Could you check a few things on this model? Use its own coordinates, in mm. A direction names the side the tool comes from. Give positions to 0.01 mm unless a question says otherwise; leave off trailing zeros. Write each loop counter-clockwise with the first axis right and the second up, starting at its lowest first coordinate (ties: lowest second). Pieces come first, ordered by that corner, then holes. Notation, with made-up numbers: M 72,3.25 L 124,3.25 A14 cw 124,28.25 Z; hole C 59.25,31.5 d3. An arc over 180 degrees is marked long. Use one line per item in the form item = value.
from build123d import *

# Parameters (mm, degrees)
SKETCH1_W           = 20.05
SKETCH1_H           = 21.2
BOSS_EXTRUDE1_DEPTH = 7
SKETCH2_W           = 20.05
SKETCH2_H           = 21.2
BOSS_EXTRUDE2_DEPTH = 1
SKETCH3_W           = 20.05
SKETCH3_H           = 11.7
BOSS_EXTRUDE3_DEPTH = 7
SKETCH4_W           = 20.05
SKETCH4_H           = 11.7
BOSS_EXTRUDE4_DEPTH = 1
BOSS_EXTRUDE5_DEPTH = 20.05
BOSS_EXTRUDE6_DEPTH = 1
BOSS_EXTRUDE7_DEPTH = 1


with BuildPart() as part:
    # Sketch1 → Boss-Extrude1 (new body)
    with BuildSketch(Plane.XY):
        with Locations((1.45, 4.75)):
            Rectangle(SKETCH1_W, SKETCH1_H)
        with BuildLine():
            Line((-5.975, 3.85), (6.51326417, 3.85))
            Line((6.51326417, 3.85), (9.475, 1.194650635))
            Line((9.475, 1.194650635), (9.475, 0.75))
            Line((9.475, 0.75), (9.875, 0.75))
            Line((9.875, 0.75), (9.875, -0.75))
            Line((9.875, -0.75), (9.475, -0.75))
            Line((9.475, -0.75), (9.475, -1.194650635))
            Line((9.475, -1.194650635), (6.51326417, -3.85))
            Line((6.51326417, -3.85), (-5.975, -3.85))
            ThreePointArc((-5.975, -3.85), (-6.399264069, -3.674264069), (-6.575, -3.25))
            Line((-6.575, -3.25), (-6.575, -0.75))
            Line((-6.575, -0.75), (-6.975, -0.75))
            Line((-6.975, -0.75), (-6.975, 0.75))
            Line((-6.975, 0.75), (-6.575, 0.75))
            Line((-6.575, 0.75), (-6.575, 3.25))
            ThreePointArc((-6.575, 3.25), (-6.399264069, 3.674264069), (-5.975, 3.85))
        make_face(mode=Mode.SUBTRACT)
        with BuildLine():
            Line((-5.975, 13.35), (6.51326417, 13.35))
            Line((6.51326417, 13.35), (9.475, 10.694650635))
            Line((9.475, 10.694650635), (9.475, 10.25))
            Line((9.475, 10.25), (9.875, 10.25))
            Line((9.875, 10.25), (9.875, 8.75))
            Line((9.875, 8.75), (9.475, 8.75))
            Line((9.475, 8.75), (9.475, 8.305349365))
            Line((9.475, 8.305349365), (6.51326417, 5.65))
            Line((6.51326417, 5.65), (-5.975, 5.65))
            ThreePointArc((-5.975, 5.65), (-6.399264069, 5.825735931), (-6.575, 6.25))
            Line((-6.575, 6.25), (-6.575, 8.75))
            Line((-6.575, 8.75), (-6.975, 8.75))
            Line((-6.975, 8.75), (-6.975, 10.25))
            Line((-6.975, 10.25), (-6.575, 10.25))
            Line((-6.575, 10.25), (-6.575, 12.75))
            ThreePointArc((-6.575, 12.75), (-6.399264069, 13.174264069), (-5.975, 13.35))
        make_face(mode=Mode.SUBTRACT)
    extrude(amount=-BOSS_EXTRUDE1_DEPTH)

    # Sketch2 → Boss-Extrude2 (add)
    with BuildSketch(Plane.XY):
        with Locations((1.45, 4.75)):
            Rectangle(SKETCH2_W, SKETCH2_H)
        Polygon((6.0923583, 2.75), (-5.475, 2.75), (-5.475, -2.75), (6.0923583, -2.75), (8.375, -0.703493649), (8.375, 0.703493649), align=None, mode=Mode.SUBTRACT)
        Polygon((6.0923583, 12.25), (-5.475, 12.25), (-5.475, 6.75), (6.0923583, 6.75), (8.375, 8.796506351), (8.375, 10.203493649), align=None, mode=Mode.SUBTRACT)
    extrude(amount=BOSS_EXTRUDE2_DEPTH)



with BuildPart() as body_2:
    # Sketch3 → Boss-Extrude3 (new body)
    with BuildSketch(Plane(origin=(0, 0, 11), x_dir=(-1, 0, 0), z_dir=(0, 0, -1))):
        with Locations((-1.45, 4.75)):
            Rectangle(SKETCH3_W, SKETCH3_H)
        with BuildLine():
            Line((6.975, 4), (6.575, 4))
            Line((6.575, 4), (6.575, 1.5))
            ThreePointArc((6.575, 1.5), (6.399264069, 1.075735931), (5.975, 0.9))
            Line((5.975, 0.9), (-6.51326417, 0.9))
            Line((-6.51326417, 0.9), (-9.475, 3.555349365))
            Line((-9.475, 3.555349365), (-9.475, 4))
            Line((-9.475, 4), (-9.875, 4))
            Line((-9.875, 4), (-9.875, 5.5))
            Line((-9.875, 5.5), (-9.475, 5.5))
            Line((-9.475, 5.5), (-9.475, 5.944650635))
            Line((-9.475, 5.944650635), (-6.51326417, 8.6))
            Line((-6.51326417, 8.6), (5.975, 8.6))
            ThreePointArc((5.975, 8.6), (6.399264069, 8.424264069), (6.575, 8))
            Line((6.575, 8), (6.575, 5.5))
            Line((6.575, 5.5), (6.975, 5.5))
            Line((6.975, 5.5), (6.975, 4))
        make_face(mode=Mode.SUBTRACT)
    extrude(amount=-BOSS_EXTRUDE3_DEPTH)

    # Sketch4 → Boss-Extrude4 (add)
    with BuildSketch(Plane(origin=(0, 0, 11), x_dir=(-1, 0, 0), z_dir=(0, 0, -1))):
        with Locations((-1.45, 4.75)):
            Rectangle(SKETCH4_W, SKETCH4_H)
        Polygon((-6.0923583, 2), (5.475, 2), (5.475, 7.5), (-6.0923583, 7.5), (-8.375, 5.453493649), (-8.375, 4.046506351), align=None, mode=Mode.SUBTRACT)
    extrude(amount=BOSS_EXTRUDE4_DEPTH)


with BuildPart() as part_1:
    add(part.part)

    add(body_2.part)  # Boss-Extrude5 merges body 2
    # Sketch5 → Boss-Extrude5 (add)
    with BuildSketch(Plane(origin=(11.475, 0, 0), x_dir=(0, 0, -1), z_dir=(1, 0, 0))):
        Polygon((-10, -1.1), (-1, -5.85), (-1, -4.85), (-10, -0.1), align=None)
        Polygon((-10, 9.6), (-1, 14.35), (-1, 15.35), (-10, 10.6), align=None)
    extrude(amount=-BOSS_EXTRUDE5_DEPTH)

    # Sketch6 → Boss-Extrude6 (add)
    with BuildSketch(Plane(origin=(11.475, 0, 0), x_dir=(0, 0, -1), z_dir=(1, 0, 0))):
        Polygon((-10, 9.6), (-1, 14.35), (-1, -4.85), (-10, -0.1), align=None)
    extrude(amount=-BOSS_EXTRUDE6_DEPTH)

    # Sketch7 → Boss-Extrude7 (add)
    with BuildSketch(Plane.ZY.offset(8.575)):
        Polygon((1, -4.85), (1, 14.35), (10, 9.6), (10, -0.1), align=None)
    extrude(amount=-BOSS_EXTRUDE7_DEPTH)


solid = part_1.part
1) I want a section at B-B, the plane y = 13.75. Please give me the cut outline in (x, z) (3 decimals), plus the area to 3 significant figures.
Checked values:
outline = M -8.575,-7 L 11.475,-7 L 11.475,4.032 L -8.575,4.032 Z; hole M -7.575,1 L 10.475,1 L 10.475,2.137 L -7.575,2.137 Z
area = 201 mm2
2) I want a section at A-A, the plane z = 16.25. Please give me the cut outline in (x, y) (3 decimals), plus the area to 3 significant figures.
Checked values:
outline = M -8.575,-1.1 L 11.475,-1.1 L 11.475,10.6 L -8.575,10.6 Z; hole M -6.975,4 L -6.575,4 L -6.575,1.5 A0.6 ccw -5.975,0.9 L 6.513,0.9 L 9.475,3.555 L 9.475,4 L 9.875,4 L 9.875,5.5 L 9.475,5.5 L 9.475,5.945 L 6.513,8.6 L -5.975,8.6 A0.6 ccw -6.575,8 L -6.575,5.5 L -6.975,5.5 Z
area = 118 mm2
3) I want a section at C-C, the plane x = 2.75. Count the separate pieces of the cut face and the enclosed holes in it, plus the area to 3 significant figures.
Checked values:
separate_pieces = 3
enclosed_holes = 0
area = 103 mm2
4) I want a section at D-D, the plane y = 9.25. Please give me the cut outline in (x, z) (3 decimals), plus the area to 3 significant figures.
Checked values:
outline = M -8.575,-7 L -6.975,-7 L -6.975,0 L -5.475,0 L -5.475,1 L -7.575,1 L -7.575,10 L 10.475,10 L 10.475,1 L 8.375,1 L 8.375,0 L 9.875,0 L 9.875,-7 L 11.475,-7 L 11.475,18 L -8.575,18 Z
area = 207 mm2
5) For faces 3 (the flat face through (-6.975, 0, -3)), 4 (the flat face through (2, 10.6, 14)), 5 (the flat face through (8.375, 4.8, 10.5)), which set-ups out of +Z, -Z, +X, -X, +Y, -Y let a thin tool reach every point of the face, with its end or its side?
Checked values:
face_3 = -Z
face_4 = +Z, +X, -X, +Y
face_5 = +Z
6) If I drill on L1, parallel to Y at x = -1.75, z = -3; L2, parallel to X at y = 3.75, z = 7.25 (3 decimals); L3, parallel to Z at x = 2.75, y = 3.5, over which ranges is the centre line in solid material (lowest first)?
Checked values:
L1 = -5.85 to -3.85, 3.85 to 5.65, 13.35 to 15.35
L2 = -8.575 to -7.575, 10.475 to 11.475
L3 = 0 to 1
7) For pin 1 Ø4 at (x, z) = (-1.5, 13.5) entering from -Y; pin 2 Ø10 at (x, y) = (4, -3.5) entering from -Z; pin 3 Ø12 at (x, z) = (-4, 13.5) entering from +Y; pin 4 Ø0.5 at (x, z) = (2.5, 10.5) entering from +Y, each with a flat end and sliding along its axis, tell me the tip position at first contact or that it passes through.
Checked values:
pin_1 = -1.1
pin_2 = -7
pin_3 = 11.92
pin_4 = 10.6
8) Thinking about a two-plate mould opening in X: for faces 1 (the flat face through (1, -5.85, -3)), 2 (the flat face through (-5.475, 9.5, 0.5)), which applies, released by +X, released by -X, zero draft, split by the parting line, or undercut?
Checked values:
face_1 = zero draft
face_2 = undercut
